Autodesk Inventor part; units mm, degrees
ref_plane "YZ Plane" through (0, 0, 0) normal (1, 0, 0) x (0, 1, 0)
ref_plane "XZ Plane" through (0, 0, 0) normal (0, 1, 0) x (-1, 0, 0)
ref_plane "XY Plane" through (0, 0, 0) normal (0, 0, 1) x (1, 0, 0)
sketch "Sketch1" plane through (0, 0, 0) normal (0, 0, 1) x (1, 0, 0)
  circle A0 centre (0, 0) radius 13.25
  circle A1 centre (0, 8.5) radius 2.125
  circle A2 centre (0, 0) radius 2.125
  circle A3 centre (0, 0) radius 4.25
  circle A4 centre (-7.3612, -4.25) radius 2.125
  circle A5 centre (7.3612, -4.25) radius 2.125
  dimension "d0" = 26.5
  dimension "d1" = 4.25
  dimension "d2" = 8.5
  dimension "d3" = 0
  dimension "d4" = 4.25
  dimension "d5" = 8.5
  dimension "d8" = 360
extrude "Extrusion1" add sketch "Sketch1" along normal blind 4.25 contours A0 | A3
extrude "Extrusion2" add sketch "Sketch1" along normal blind 13 contours A3
equation "\"d4\" = d1"
equation "\"d5\" = 2 * d1"
equation "\"d10\" = d1"
The model under review builds one solid part; all positions refer to its coordinate system, in mm. A direction names the side the tool comes from. Coordinates: 2 decimals unless noted, no trailing zeros. Write each loop counter-clockwise with the first axis right and the second up, starting at its lowest first coordinate (ties: lowest second). Pieces come first, ordered by that corner, then holes. Notation, with made-up numbers: M 32.5,38 L 82.5,38 A19 cw 82.5,68 Z; hole C -6.75,30 d1. An arc over 180 degrees is marked long. Put each result on its own line as item: value.
1) Clearance check with flat-ended pins moving along their axes: pin 1 Ø7 at (x, y) = (7.36, -4.25) entering from +Z; pin 2 Ø2.5 at (x, y) = (0, 8.5) entering from +Z; pin 3 Ø1 at (x, y) = (-5, 5) entering from -Z. State where each tip first meets the part, or that it passes through.
Computed:
pin 1: stops at z = 4.25
pin 2: passes through
pin 3: stops at z = 0
2) Wall thickness on probe 1 along Y at (x, z) = (0, 5) (3 decimals); probe 2 along Y at (x, z) = (-0.5, 3.75); probe 3 along Y at (x, z) = (-1.75, 4): over which ranges is each line inside the solid? List them lowest first. Write a range as [from, to].
Computed:
probe 1: y = [-4.25, -2.125], [2.125, 4.25]
probe 2: y = [-13.24, -2.07], [2.07, 6.43], [10.57, 13.24]
probe 3: y = [-13.13, -1.21], [1.21, 7.29], [9.71, 13.13]
3) Draft analysis for pull direction Y (two halves, no side actions). For faces 3 (the flat face through (2, -2, 13)), 4 (the cylindrical face through (7.123, -11.172, 2.095)), 5 (the cylindrical face through (5.675, -2.957, 2.095)), state which applies: released by +Y, released by -Y, zero draft, split by the parting line, or undercut.
Computed:
face 3: zero draft
face 4: split by the parting line
face 5: undercut
4) Add section B-B on y = 0. Give the boundary of the cut face in (x, z) (3 decimals), then the cut area to 3 significant figures.
Computed:
outline: M -13.25,0 L -2.125,0 L -2.125,13 L -4.25,13 L -4.25,4.25 L -13.25,4.25 Z; M 2.125,0 L 13.25,0 L 13.25,4.25 L 4.25,4.25 L 4.25,13 L 2.125,13 Z
area: 132 mm2
5) For faces 1 (the flat face through (-3.13, 3.13, 4.25)), 2 (the cylindrical face through (-0.461, 10.574, 2.095)), list the 3-axis set-ups (+Z, -Z, +X, -X, +Y, -Y) from which the entire face can be reached by the end or side of a thin tool; tool diameter is ignored.
Computed:
face 1: +Z
face 2: +Z, -Z
6) Add section A-A on x = 0. Give the boundary of the cut face in (y, z) (3 decimals), then the cut area to 3 significant figures.
Computed:
outline: M -13.25,0 L -2.125,0 L -2.125,13 L -4.25,13 L -4.25,4.25 L -13.25,4.25 Z; M 2.125,0 L 6.375,0 L 6.375,4.25 L 4.25,4.25 L 4.25,13 L 2.125,13 Z; M 10.625,0 L 13.25,0 L 13.25,4.25 L 10.625,4.25 Z
area: 114 mm2
7) Add section D-D on x = 9. Give the boundary of the cut face in (y, z), then the cut area to 3 significant figures.
Computed:
outline: M -9.72,0 L -5.6,0 L -5.6,4.25 L -9.72,4.25 Z; M -2.9,0 L 9.72,0 L 9.72,4.25 L -2.9,4.25 Z
area: 71.2 mm2
8) Add section C-C on z = 7.75. Give the boundary of the cut face in (x, y) (3 decimals).
Computed:
outline: C 0,0 d8.5; hole C 0,0 d4.25
